Autodesk Inventor part; units mm, degrees
ref_plane "YZ Plane" through (0, 0, 0) normal (1, 0, 0) x (0, 1, 0)
ref_plane "XZ Plane" through (0, 0, 0) normal (0, 1, 0) x (-1, 0, 0)
ref_plane "XY Plane" through (0, 0, 0) normal (0, 0, 1) x (1, 0, 0)
sketch "Sketch1" plane through (0, 0, 0) normal (0, 1, 0) x (-1, 0, 0)
  line L0 (0, 0) -> (110, 0)
  line L1 (110, 0) -> (110, -100)
  line L2 (110, -100) -> (0, -100)
  line L3 (0, -100) -> (0, 0)
  dimension "d0" = 110
  dimension "d1" = 100
extrude "Extrusion1" add sketch "Sketch1" along normal blind 5
sketch "Sketch2" plane through (0, 5, 0) normal (0, 1, 0) x (1, 0, 0)
  point P0 (0, 0)
sketch "Sketch3" plane through (0, 0, 0) normal (0, -1, 0) x (1, 0, 0)
  circle A0 centre (-4, -2.5) radius 1.5
  point P0 (0, 0)
  dimension "d4" = 3
extrude "Extrusion2" add sketch "Sketch3" along normal blind 1.5
sketch "Sketch4" plane through (-4, -1.5, -2.5) normal (0, -1, 0) x (1, 0, 0)
  point P0 (4, 2.5)
sketch "Sketch5" plane through (-4, -1.5, -2.5) normal (0, -1, 0) x (1, 0, 0)
  line L0 (1.5, 0.5) -> (-1.5, 0.5)
  line L1 (-1.5, 0.5) -> (-1.5, -0.5)
  line L2 (-1.5, -0.5) -> (1.5, -0.5)
  line L3 (1.5, -0.5) -> (1.5, 0.5)
  line L4 (1.5, 0.5) -> (-1.5, -0.5) construction
  line L5 (-1.5, 0.5) -> (1.5, -0.5) construction
  point P0 (4, 2.5)
  point P1 (0, 0)
  dimension "d7" = 1
extrude "Extrusion3" cut sketch "Sketch5" against normal blind 1
pattern_linear "Rectangular Pattern1" count 2 spacing 100 along (-1, 0, 0) of "Extrusion3", "Extrusion2"
pattern_linear "Rectangular Pattern2" count 2 spacing 95 along (0, 0, -1) of "Extrusion2", "Extrusion3"
pattern_linear "Rectangular Pattern3" count 2 spacing 95 along (0, 0, -1) of "Extrusion3", "Extrusion2", "Rectangular Pattern1"
properties part number "bottom part"
Check sheet for the modelled part. Datum: model origin and axes. Units: mm. A direction names the side the tool comes from. Round coordinates to 2 decimals unless told otherwise and drop trailing zeros. Write each loop counter-clockwise with the first axis right and the second up, starting at its lowest first coordinate (ties: lowest second). Pieces come first, ordered by that corner, then holes. Notation, with made-up numbers: (2, 1) -> (18, 1) arc R15 cw to (18, 23) -> close; hole circle Ø6 at (-0.5, -35). An arc over 180 degrees is marked (long way). Put each result on its own line as item: value.
(1) Sectioned sample at C-C (x = -95). Enter the section's corners in (y, z).
Values found:
outline: (0, -100) -> (5, -100) -> (5, 0) -> (0, 0) -> close
(2) Sectioned sample at A-A (x = -4). Enter the section's corners in (y, z), plus the area to 3 significant figures.
Values found:
outline: (-1.5, -99) -> (0, -99) -> (0, -100) -> (5, -100) -> (5, 0) -> (0, 0) -> (0, -1) -> (-1.5, -1) -> (-1.5, -2) -> (-0.5, -2) -> (-0.5, -3) -> (-1.5, -3) -> (-1.5, -4) -> (0, -4) -> (0, -96) -> (-1.5, -96) -> (-1.5, -97) -> (-0.5, -97) -> (-0.5, -98) -> (-1.5, -98) -> close
area: 507 mm^2
(3) Material ranges on line 1 (Y direction, x = -71, z = -60.5), recorded low to high.
Values found:
line 1: y = 0 to 5
(4) Sectioned sample at B-B (z = -64.5). Enter the section's corners in (x, y), plus the area to 3 significant figures.
Values found:
outline: (-110, 0) -> (0, 0) -> (0, 5) -> (-110, 5) -> close
area: 550 mm^2
(5) Tool access check on faces 1 (the face through (-103.31, -0.74, -1.17)), 2 (the face through (-54, 2, 0)). Record the directions out of +Z, -Z, +X, -X, +Y, -Y that give a thin tool (end or side, any length) a straight path to the whole face; none if there is none.
Values found:
face 1: -Y
face 2: +Z, +X, -X, +Y, -Y
(6) Go/stop test with flat-tipped pins: pin 1 Ø6 at (x, z) = (-58, -28) entering from -Y; pin 2 Ø1.1 at (x, y) = (-104, -1) entering from +Z; pin 3 Ø0.5 at (x, y) = (-4.5, -1) entering from -Z. Record where each tip stops, or that it passes through.
Values found:
pin 1: stops at y = 0
pin 2: stops at z = -1
pin 3: stops at z = -98.98
(7) Mould release check, pull along Z, two halves, no side actions. Record for faces 3 (the face through (-54, 5, -49)), 4 (the face through (-56, 2, -100)), 5 (the face through (-103.31, -0.74, -96.17)): released by +Z, released by -Z, zero draft, split by the parting line, or undercut.
Values found:
face 3: zero draft
face 4: released by -Z
face 5: undercut
